Part model, mm, in its own coordinate system. A direction names the side the tool comes from. Coordinates: 2 decimals unless noted, no trailing zeros. Order: outer loops, then holes, each group sorted by start corner. A loop starts at its lowest first (then second) coordinate and runs counter-clockwise, first axis right, second up. Notation, with made-up numbers: M 68.25,78.25 L 83.25,78.25 A21 ccw 83.25,95.25 Z; hole C 33.5,22.25 d4. An arc over 180 degrees is marked long. Write item = value, one per line. Start each with the question number.
from build123d import *

# Parameters (mm, degrees)
SKETCH1_W           = 83.65
SKETCH1_H           = 56
SKETCH1_R           = 1.6
BOSS_EXTRUDE1_DEPTH = 3
SKETCH2_W           = 83.65
SKETCH2_H           = 10
BOSS_EXTRUDE2_DEPTH = 70
SKETCH3_W           = 4.1
SKETCH3_H           = 3.1
CUT_EXTRUDE1_DEPTH  = 67
CHAMFER1_SIZE       = 0.1
CHAMFER2_SIZE       = 0.1
SKETCH4_R           = 1.6
CUT_EXTRUDE2_DEPTH  = 10
CUT_EXTRUDE3_START  = -3
SKETCH5_R           = 3.6
SKETCH5_R_2         = 1.6
CUT_EXTRUDE3_DEPTH  = 3


with BuildPart() as part:
    # Sketch1 → Boss-Extrude1 (new body)
    with BuildSketch(Plane(origin=(0, 0, 0), x_dir=(1, 0, 0), z_dir=(0, 1, 0))):
        Rectangle(SKETCH1_W, SKETCH1_H)
        with Locations(Location((-34.825, -21, 0), (0, 0, 270))):
            Circle(SKETCH1_R, mode=Mode.SUBTRACT)
        with Locations(Location((34.825, -21, 0), (0, 0, 270))):
            Circle(SKETCH1_R, mode=Mode.SUBTRACT)
        with Locations(Location((34.825, 21, 0), (0, 0, 270))):
            Circle(SKETCH1_R, mode=Mode.SUBTRACT)
        with Locations(Location((-34.825, 21, 0), (0, 0, 270))):
            Circle(SKETCH1_R, mode=Mode.SUBTRACT)
    extrude(amount=BOSS_EXTRUDE1_DEPTH)

    # Sketch2 → Boss-Extrude2 (add)
    with BuildSketch(Plane(origin=(0, 0, 0), x_dir=(1, 0, 0), z_dir=(0, 1, 0))):
        with Locations((0, 33)):
            Rectangle(SKETCH2_W, SKETCH2_H)
    extrude(amount=BOSS_EXTRUDE2_DEPTH)

    # Sketch3 → Cut-Extrude1 (cut)
    with BuildSketch(Plane(origin=(0, 70, 0), x_dir=(1, 0, 0), z_dir=(0, 1, 0))):
        Polygon((-3.05, 31), (-3.05, 28), (3.05, 28), (3.05, 31), (3.05, 34.1), (-3.05, 34.1), align=None)
        with Locations((-5.1, 32.55)):
            Rectangle(SKETCH3_W, SKETCH3_H)
        with Locations((5.1, 32.55)):
            Rectangle(SKETCH3_W, SKETCH3_H)
        with Locations((33.675, 32.55)):
            Rectangle(SKETCH3_W, SKETCH3_H)
        Polygon((35.725, 31), (35.725, 28), (41.825, 28), (41.825, 34.1), (35.725, 34.1), align=None)
        with Locations((-33.675, 32.55)):
            Rectangle(SKETCH3_W, SKETCH3_H)
        Polygon((-35.725, 31), (-35.725, 34.1), (-41.825, 34.1), (-41.825, 28), (-35.725, 28), align=None)
    extrude(amount=-CUT_EXTRUDE1_DEPTH, mode=Mode.SUBTRACT)

    # Chamfer1
    chamfer1_edges = [part.edges().sort_by_distance(p)[0] for p in [
        (3.05, 36.5, -31),
        (3.05, 36.5, -28),
        (-3.05, 36.5, -28),
        (-3.05, 36.5, -31),
        (35.725, 36.5, -28),
        (35.725, 36.5, -31),
        (-35.725, 36.5, -28),
        (-35.725, 36.5, -31),
    ]]
    chamfer(chamfer1_edges, length=CHAMFER1_SIZE)

    # Chamfer2
    chamfer2_edges = [part.edges().sort_by_distance(p)[0] for p in [
        (-35.725, 70, -29.5),
        (19.3875, 70, -28),
        (35.725, 70, -29.5),
        (-19.3875, 70, -28),
        (-3.05, 70, -29.5),
        (-5.15, 70, -31),
        (5.15, 70, -31),
        (3.05, 70, -29.5),
        (-3.1, 70, -28.05),
        (-3.1, 70, -30.95),
        (35.675, 70, -28.05),
        (35.675, 70, -30.95),
        (3.1, 70, -28.05),
        (3.1, 70, -30.95),
        (-35.675, 70, -30.95),
        (-35.675, 70, -28.05),
        (-41.825, 70, -36.05),
        (0, 70, -38),
        (-7.15, 70, -32.55),
        (0, 70, -34.1),
        (7.15, 70, -32.55),
        (41.825, 70, -36.05),
        (33.625, 70, -31),
        (36.725, 70, -34.1),
        (31.625, 70, -32.55),
        (-31.625, 70, -32.55),
        (-36.725, 70, -34.1),
        (-33.625, 70, -31),
    ]]
    chamfer(chamfer2_edges, length=CHAMFER2_SIZE)

    # Sketch4 → Cut-Extrude2 (cut)
    with BuildSketch(Plane(origin=(0, 0, -38), x_dir=(-1, 0, 0), z_dir=(0, 0, -1))):
        with Locations((-20, 20)):
            Circle(SKETCH4_R)
        with Locations((-20, 50)):
            Circle(SKETCH4_R)
        with Locations((20, 20)):
            Circle(SKETCH4_R)
        with Locations((20, 50)):
            Circle(SKETCH4_R)
    extrude(amount=-CUT_EXTRUDE2_DEPTH, mode=Mode.SUBTRACT)

    # Sketch5 → Cut-Extrude3 (cut)
    # profile 1 of 4: a face of its own
    with BuildSketch(Plane.XY.offset(-28).offset(CUT_EXTRUDE3_START)):
        with Locations((-20, 20)):
            Circle(SKETCH5_R)
        with Locations((-20, 20)):
            Circle(SKETCH5_R_2, mode=Mode.SUBTRACT)
    # profile 2 of 4: a face of its own
    with BuildSketch(Plane.XY.offset(-28).offset(CUT_EXTRUDE3_START)):
        with Locations((20, 20)):
            Circle(SKETCH5_R)
    # profile 3 of 4: a face of its own
    with BuildSketch(Plane.XY.offset(-28).offset(CUT_EXTRUDE3_START)):
        with Locations((20, 50)):
            Circle(SKETCH5_R)
    # profile 4 of 4: a face of its own
    with BuildSketch(Plane.XY.offset(-28).offset(CUT_EXTRUDE3_START)):
        with Locations((-20, 50)):
            Circle(SKETCH5_R)
    extrude(amount=CUT_EXTRUDE3_DEPTH, mode=Mode.SUBTRACT)


solid = part.part
Item 1: 3-axis set-ups, long thin cutter, end or side, ignore diameter. For faces 4 (the flat face through (21, 48, -31)), 5 (the flat face through (35.725, 37, -30)), 6 (the flat face through (-20, 36, -28)), 7 (the flat face through (37, 37, -34.1)), 8 (the flat face through (-7.15, 37, -33)): which of +Z, -Z, +X, -X, +Y, -Y reach the whole face in a straight line?
Item 2: Flat gauge pins, fed straight in: pin 1 (3 mm diameter, centred on y = 40, z = -29.5, fed in from +X) (3 decimals); pin 2 (12 mm diameter, centred on x = -31.5, y = 50, fed in from +Z); pin 3 (8 mm diameter, centred on x = -27, z = 6, fed in from +Y). Where does each tip first touch, or does it go through?
Item 3: Cut at B-B, the plane z = -21. Write the cut outline in (x, y) (3 decimals).
Item 4: Pull direction Z, two halves, no side cores. Call faces 1 (the flat face through (-41.825, 24, -37)), 2 (the flat face through (-18, 19, -31)), 3 (the cylindrical face through (33.406, 1.479, -20.262)): pulls with the +Z half, pulls with the -Z half, needs draft (parallel to the pull), parting line crosses it, or undercut.
Item 5: Cut at D-D, the plane y = 55. Write the cut outline in (x, z) (3 decimals), and give its area (3 significant figures).
Item 6: Cut at A-A, the plane x = 20. Write the cut outline in (y, z).
Item 7: Cut at C-C, the plane x = -27. Write the cut outline in (y, z), and give its area (3 significant figures).
Item 8: Wall check: line 1 along Y through (x, z) = (20, -34); line 2 along X through (y, z) = (1, -21) (3 decimals); line 3 along Y through (x, z) = (20, -29.1). Give the ranges that are in metal, low to high. Write a range as [from, to].
Filled sheet:
q1.face_4 = +Z
q1.face_5 = +Z, +X, +Y
q1.face_6 = +Z, +X, -X, +Y
q1.face_7 = +X, +Y
q1.face_8 = +Y
q2.pin_1 = 35.725
q2.pin_2 = -28
q2.pin_3 = 3
q3.outline = M -41.825,0 L -36.425,0 L -36.425,3 L -41.825,3 Z; M -33.225,0 L 33.225,0 L 33.225,3 L -33.225,3 Z; M 36.425,0 L 41.825,0 L 41.825,3 L 36.425,3 Z
q4.face_1 = needs draft
q4.face_2 = pulls with the +Z half
q4.face_3 = undercut
q5.outline = M -41.825,-38 L 41.825,-38 L 41.825,-34.1 L 31.625,-34.1 L 31.625,-31 L 35.625,-31 L 35.725,-30.9 L 35.725,-28.1 L 35.625,-28 L 3.15,-28 L 3.05,-28.1 L 3.05,-30.9 L 3.15,-31 L 7.15,-31 L 7.15,-34.1 L -7.15,-34.1 L -7.15,-31 L -3.15,-31 L -3.05,-30.9 L -3.05,-28.1 L -3.15,-28 L -35.625,-28 L -35.725,-28.1 L -35.725,-30.9 L -35.625,-31 L -31.625,-31 L -31.625,-34.1 L -41.825,-34.1 Z
q5.area = 674 mm2
q6.outline = M 0,-38 L 18.4,-38 L 18.4,-31 L 16.4,-31 L 16.4,-28 L 3,-28 L 3,28 L 0,28 Z; M 21.6,-38 L 48.4,-38 L 48.4,-31 L 46.4,-31 L 46.4,-28 L 23.6,-28 L 23.6,-31 L 21.6,-31 Z; M 51.6,-38 L 69.9,-38 L 70,-37.9 L 70,-28.1 L 69.9,-28 L 53.6,-28 L 53.6,-31 L 51.6,-31 Z
q7.outline = M 0,-38 L 69.9,-38 L 70,-37.9 L 70,-28.1 L 69.9,-28 L 3,-28 L 3,28 L 0,28 Z
q7.area = 868 mm2
q8.line_1 = [0, 18.4], [21.6, 48.4], [51.6, 70]
q8.line_2 = [-41.825, -36.425], [-33.225, 33.225], [36.425, 41.825]
q8.line_3 = [0, 16.4], [23.6, 46.4], [53.6, 70]
